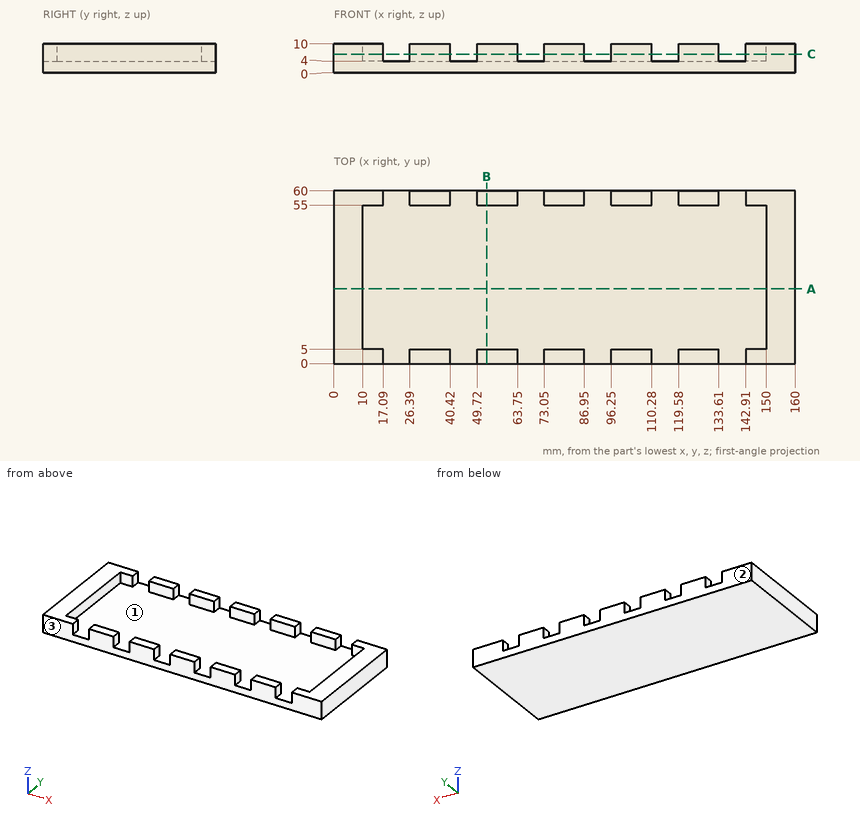
Can you work these out from the drawing? Everything is in mm from the part's minimum corner. Coordinates: 2 decimals unless noted, no trailing zeros. Loops run counter-clockwise (first coordinate to the right, second up) from the corner with the lowest first, then second, coordinate; pieces in that order, holes last.
1) Imagine slicing it at B-B (x = 53). List the corners of the cut face in (y, z) for me, and give its area (3 significant figures).
Reported:
outline: (0, 0) - (60, 0) - (60, 10) - (55, 10) - (55, 4) - (5, 4) - (5, 10) - (0, 10) - close
area: 300 mm2
2) Thinking about a two-plate mould opening in Y: for the marked faces 1, 2 and 3, which applies, released by +Y, released by -Y, zero draft, split by the parting line, or undercut?
Reported:
face 1: undercut
face 2: released by +Y
face 3: released by -Y
3) Imagine slicing it at A-A (y = 26). List the corners of the cut face in (x, z) for me.
Reported:
outline: (0, 0) - (160, 0) - (160, 10) - (150, 10) - (150, 4) - (10, 4) - (10, 10) - (0, 10) - close
4) Imagine slicing it at C-C (z = 6.5). State how many separate pieces and enclosed holes the cut face has, and give its area (3 significant figures).
Reported:
separate pieces: 12
enclosed holes: 0
area: 2,040 mm2
5) Please list where these lines run through material, in increasing order: line 1 along X through (y, z) = (45.5, 8.25); line 2 along Y through (x, z) = (147.5, 7.5); line 3 along Z through (x, y) = (27, 10.5).
Reported:
line 1: x = 0 to 10, 150 to 160
line 2: y = 0 to 5, 55 to 60
line 3: z = 0 to 4
